Autodesk Inventor part; units mm, degrees
ref_plane "YZ Plane" through (0, 0, 0) normal (1, 0, 0) x (0, 1, 0)
ref_plane "XZ Plane" through (0, 0, 0) normal (0, 1, 0) x (-1, 0, 0)
ref_plane "XY Plane" through (0, 0, 0) normal (0, 0, 1) x (1, 0, 0)
sketch "Sketch1" plane through (0, 0, 0) normal (0, 1, 0) x (-1, 0, 0)
  line L0 (0, 0) -> (38.608, 0)
  line L1 (38.608, 0) -> (38.608, -38.608)
  line L2 (38.608, -38.608) -> (0, -38.608)
  line L3 (0, -38.608) -> (0, 0)
  dimension "d0" = 38.608
  dimension "d1" = 38.608
extrude "Extrusion1" add sketch "Sketch1" along normal blind 5.08
sketch "Sketch2" plane through (0, 0, 0) normal (0, -1, 0) x (1, 0, 0)
  line L0 (-38.608, 0) -> (0, 0)
  circle A0 centre (-19.304, -19.304) radius 15.875
  line L1 (-38.608, -38.608) -> (-38.608, 0)
  line L2 (-38.608, -19.304) -> (-38.608, -21.082)
  line L3 (-38.608, -21.082) -> (-34.9151, -21.082)
  line L4 (-34.9151, -21.082) -> (-34.9151, -16.4216)
  line L5 (-34.9151, -16.4216) -> (-38.608, -16.4216)
  line L6 (-38.608, -16.4216) -> (-38.608, -21.082)
  line L7 (-19.304, -19.304) -> (-19.304, -38.608)
  line L8 (0, -38.608) -> (-38.608, -38.608)
  line L9 (-12.192, -31.75) -> (-12.192, -38.608)
  line L10 (-12.192, -38.608) -> (-26.416, -38.608)
  line L11 (-26.416, -38.608) -> (-26.416, -31.75)
  line L12 (-26.416, -31.75) -> (-12.192, -31.75)
  line L13 (-12.192, -31.75) -> (-26.416, -38.608) construction
  line L14 (-12.192, -38.608) -> (-26.416, -31.75) construction
  line L15 (-19.304, -19.304) -> (-0.2032, -19.304) construction
  circle A1 centre (-31.8453, -4.8972) radius 4.318
  point P0 (-35.0791, -21.082)
  point P1 (-19.304, -35.179)
  point P2 (-26.416, -33.4968)
  point P3 (-12.192, -33.4968)
  point P4 (-31.5527, -9.2053)
  point P5 (-27.6186, -5.7806)
  dimension "d4" = 31.75
  dimension "d8" = 14.224
  dimension "d11" = 8.636
  dimension "d42" = 6.858
  dimension "d43" = 3.6929
  dimension "d44" = 4.6604
  dimension "d45" = 3.6929
extrude "Extrusion2" cut sketch "Sketch2" against normal blind 6.35 contours A0 L9 L12 L11 L3 L4 A1 | A1 A0 | A0 A1 | L9 L8 L7 A0 | A0 L7 L12 L9 | L7 L8 L11 A0 | A0 L11 L12 L7 | L4 L3 A0 | A0 L3 L1 L5
sketch "Sketch4" plane through (0, 0, 0) normal (1, 0, 0) x (0, 0, -1)
  line L0 (38.608, 0) -> (38.608, 5.08)
  line L1 (0, 5.08) -> (38.608, 5.08)
  line L2 (12.954, 6.35) -> (25.654, 6.35)
  line L3 (14.224, 0) -> (14.224, 6.35)
  line L4 (14.224, 6.35) -> (24.384, 6.35)
  line L5 (24.384, 6.35) -> (24.384, 0)
  line L6 (24.384, 0) -> (14.224, 0)
  line L7 (14.224, 0) -> (24.384, 6.35) construction
  line L8 (14.224, 6.35) -> (24.384, 0) construction
  point P0 (0, 0)
  point P1 (19.304, 3.175)
  point P2 (24.384, 5.08)
  point P3 (14.224, 5.08)
  dimension "d19" = 10.16
extrude "Extrusion4" add sketch "Sketch4" along normal blind 38.1 contours L1 L5 L6 L3
sketch "Sketch6" plane through (-38.608, 0, 0) normal (0, 0, 1) x (1, 0, 0)
  line L0 (0, 0) -> (3.6929, 0)
  line L1 (38.608, 5.08) -> (76.708, 5.08)
  line L2 (0, 0) -> (0, 5.08)
  line L3 (38.608, 0) -> (76.708, 0)
  line L4 (0, 5.08) -> (38.608, 5.08)
  line L5 (24.384, 5.08) -> (14.224, 5.08)
  line L6 (0, 0) -> (38.608, 0)
  line L7 (14.224, 0) -> (24.384, 0)
  line L8 (24.384, 0) -> (24.384, 5.08)
  line L9 (24.384, 5.08) -> (14.224, 5.08)
  line L10 (14.224, 5.08) -> (14.224, 0)
  line L11 (14.224, 0) -> (24.384, 5.08) construction
  line L12 (24.384, 0) -> (14.224, 5.08) construction
  point P0 (19.304, 2.54)
  dimension "d24" = 10.16
sketch "Sketch7" plane through (-38.608, 0, -38.608) normal (-1, 0, 0) x (0, 0, 1)
  line L0 (0, 0) -> (0, 5.08)
  line L1 (22.1864, 0) -> (38.608, 0)
  line L2 (22.1864, 5.08) -> (38.608, 5.08)
  line L3 (38.608, 0) -> (38.608, 5.08)
  line L4 (5.1112, 5.08) -> (35.179, 5.08)
  line L5 (24.384, 0) -> (14.224, 0)
  line L6 (14.224, 0) -> (14.224, 5.08)
  line L7 (14.224, 5.08) -> (24.384, 5.08)
  line L8 (24.384, 5.08) -> (24.384, 0)
  line L9 (24.384, 0) -> (14.224, 5.08) construction
  line L10 (14.224, 0) -> (24.384, 5.08) construction
  point P0 (32.8274, 5.08)
  point P1 (19.304, 2.54)
  dimension "d25" = 10.16
extrude "Extrusion5" add sketch "Sketch6" along normal blind 38.1 contours L10 L4 L8 L6
extrude "Extrusion6" add sketch "Sketch7" along normal blind 38.1 contours L5 L6 L4 L2 L8 L1
sketch "Sketch8" plane through (0, 0, -38.608) normal (0, 0, -1) x (-1, 0, 0)
  line L0 (0, 0) -> (0, 5.08)
  line L1 (38.608, 0) -> (34.9151, 0)
  line L2 (0, 5.08) -> (38.608, 5.08)
  line L3 (38.608, 5.08) -> (38.608, 0)
  line L4 (38.608, 0) -> (0, 0)
  line L5 (0, 0) -> (0, 5.08)
extrude "Extrusion7" add sketch "Sketch8" along normal blind 3.81
sketch "Sketch9" plane through (0, 0, -42.418) normal (0, 0, -1) x (-1, 0, 0)
  line L0 (38.608, 5.08) -> (0, 5.08)
  line L1 (38.608, 0) -> (76.708, 0)
  line L2 (3.429, 5.08) -> (27.6186, 5.08)
  line L3 (14.224, 0) -> (24.384, 0)
  line L4 (24.384, 0) -> (24.384, 5.08)
  line L5 (24.384, 5.08) -> (14.224, 5.08)
  line L6 (14.224, 5.08) -> (14.224, 0)
  line L7 (14.224, 0) -> (24.384, 5.08) construction
  line L8 (24.384, 0) -> (14.224, 5.08) construction
  point P0 (0, 0)
  point P1 (12.192, 5.08)
  point P2 (19.304, 2.54)
  point P3 (14.224, 5.08)
  dimension "d32" = 10.16
extrude "Extrusion8" add sketch "Sketch9" along normal blind 34.29
sketch "Sketch10" plane through (0, 5.08, 0) normal (0, 1, 0) x (1, 0, 0)
  line L0 (-76.708, 24.384) -> (-76.708, 14.224)
  line L1 (-38.608, 24.384) -> (-76.708, 24.384)
  line L2 (-76.708, 14.224) -> (-69.088, 14.224)
  line L3 (-69.088, 14.224) -> (-69.088, 24.384)
  line L4 (-69.088, 24.384) -> (-76.708, 24.384)
  line L5 (-76.708, 24.384) -> (-76.708, 14.224)
  line L6 (-14.224, 76.708) -> (-24.384, 76.708)
  line L7 (-14.224, 76.708) -> (-24.384, 76.708)
  line L8 (-24.384, 76.708) -> (-24.384, 69.088)
  line L9 (-24.384, 69.088) -> (-14.224, 69.088)
  line L10 (-14.224, 69.088) -> (-14.224, 76.708)
  line L11 (38.1, 14.224) -> (38.1, 24.384)
  line L12 (0, 24.384) -> (38.1, 24.384)
  line L13 (38.1, 14.224) -> (30.48, 14.224)
  line L14 (30.48, 14.224) -> (30.48, 24.384)
  line L15 (30.48, 24.384) -> (38.1, 24.384)
  line L16 (38.1, 24.384) -> (38.1, 14.224)
  line L17 (-14.224, 0) -> (-14.224, -38.1)
  line L18 (-24.384, 0) -> (-24.384, -38.1)
  line L19 (-14.224, -38.1) -> (-24.384, -38.1)
  line L20 (-24.384, -38.1) -> (-24.384, -30.48)
  line L21 (-24.384, -30.48) -> (-14.224, -30.48)
  line L22 (-14.224, -30.48) -> (-14.224, -38.1)
  point P0 (0, 0)
  dimension "d35" = 7.62
  dimension "d36" = 10.16
  dimension "d37" = 7.62
  dimension "d38" = 7.62
  dimension "d39" = 7.62
extrude "Extrusion9" add sketch "Sketch10" along normal blind 83.82
properties part number "Camera Stand 2.0"
Check sheet for the modelled part. Datum: model origin and axes. Units: mm. A direction names the side the tool comes from. Give positions to 0.01 mm unless a question says otherwise; leave off trailing zeros. Order: outer loops, then holes, each group sorted by start corner. A loop starts at its lowest first (then second) coordinate and runs counter-clockwise, first axis right, second up. Notation, with made-up numbers: (-22.5, -14.75) -> (36.5, -14.75) arc R19 cw to (36.5, 21.25) -> close; hole circle Ø9 at (-34.75, 30). An arc over 180 degrees is marked (long way). Return JSON: item names as keys, results as strings.
1. Cross-section at C-C, the plane z = -29.5. Record the cut outline in (x, y).
From the geometry:
{"outline": "(-38.61, 0) -> (-31.47, 0) -> (-31.47, 5.08) -> (-38.61, 5.08) -> close; (-7.14, 0) -> (0, 0) -> (0, 5.08) -> (-7.14, 5.08) -> close"}
2. Go/stop test with flat-tipped pins: P1, Ø2.5, axis at y = 2.5, z = -31, coming from the +X side; P2, Ø3, axis at y = 40.5, z = -12, coming from the +X side; P3, Ø5.5, axis at x = -4.5, y = 3.5, coming from the -Z side; P4, Ø1.5, axis at x = -35, y = 3, coming from the +Z side. Record where each tip stops, or that it passes through.
From the geometry:
{"P1": "x = 0", "P2": "through", "P3": "z = -42.42", "P4": "z = 0"}
3. Material ranges on probe 1 along Z at (x, y) = (-14.5, 40.5); probe 2 along Y at (x, z) = (-23, -48), recorded low to high. Write a range as [from, to].
From the geometry:
{"probe 1": "[-76.71, -69.09], [30.48, 38.1]", "probe 2": "[0, 5.08]"}
4. Set-up check for faces 5 (the flat face through (-31, 3, -42.418)), 6 (the flat face through (-24.384, 38, 33)), 7 (the flat face through (-69.088, 46, -19)): record each of +Z, -Z, +X, -X, +Y, -Y from which the full face is reachable in a straight line by a thin tool's end or side.
From the geometry:
{"face 5": "-Z, -X, +Y, -Y", "face 6": "+Z, -X, +Y, -Y", "face 7": "+Z, -Z, +Y"}
5. Cross-section at B-B, the plane x = -21. Record the cut outline in (y, z), plus the area to 3 significant figures.
From the geometry:
{"outline": "(0, -76.71) -> (88.9, -76.71) -> (88.9, -69.09) -> (5.08, -69.09) -> (5.08, -38.61) -> (0, -38.61) -> close; (0, -3.52) -> (5.08, -3.52) -> (5.08, 30.48) -> (88.9, 30.48) -> (88.9, 38.1) -> (0, 38.1) -> close", "area": "1,680 mm^2"}
6. Mould release check, pull along Z, two halves, no side actions. Record for faces 1 (the flat face through (-37, 3, -21.082)), 2 (the flat face through (-38.608, 3, -7)), 3 (the flat face through (-19, 45, -76.708)), 4 (the flat face through (-37, 3, -16.422)): +Z half, -Z half, draft (parallel to the pull), parting line (faces both ways), or undercut.
From the geometry:
{"face 1": "undercut", "face 2": "draft", "face 3": "-Z half", "face 4": "undercut"}
7. Cross-section at D-D, the plane x = -42. Record the cut outline in (y, z), plus the area to 3 significant figures.
From the geometry:
{"outline": "(0, -24.38) -> (5.08, -24.38) -> (5.08, -14.22) -> (0, -14.22) -> close", "area": "51.6 mm^2"}
8. Cross-section at A-A, the plane y = 13.5. Record the cut outline in (x, z).
From the geometry:
{"outline": "(-76.71, -24.38) -> (-69.09, -24.38) -> (-69.09, -14.22) -> (-76.71, -14.22) -> close; (-24.38, -76.71) -> (-14.22, -76.71) -> (-14.22, -69.09) -> (-24.38, -69.09) -> close; (-24.38, 30.48) -> (-14.22, 30.48) -> (-14.22, 38.1) -> (-24.38, 38.1) -> close; (30.48, -24.38) -> (38.1, -24.38) -> (38.1, -14.22) -> (30.48, -14.22) -> close"}
